Verification items for the finished model (mm, model axes). Give positions to 0.01 mm unless a question says otherwise; leave off trailing zeros. Order: outer loops, then holes, each group sorted by start corner. A loop starts at its lowest first (then second) coordinate and runs counter-clockwise, first axis right, second up.
from build123d import *

# Parameters (mm, degrees)
SKETCH001_W  = 54
SKETCH001_H  = 78
PAD001_DEPTH = 12
FILLET_R     = 2
FILLET001_R  = 2
SKETCH002_R  = 2
POCKET_DEPTH = 6
FILLET002_R  = 2


with BuildPart() as part:
    # Sketch001 (on Face1 of CopyCut) → Pad001 (new body)
    with BuildSketch(Plane.XY.offset(-3)):
        with Locations((0, 47)):
            Rectangle(SKETCH001_W, SKETCH001_H)
    extrude(amount=PAD001_DEPTH)

    # Fillet
    fillet_edges = [part.edges().sort_by_distance(p)[0] for p in [
        (0, 86, 9),
    ]]
    fillet(fillet_edges, radius=FILLET_R)

    # Fillet001
    fillet001_edges = [part.edges().sort_by_distance(p)[0] for p in [
        (-27, 46, 9),
        (27, 46, 9),
    ]]
    fillet(fillet001_edges, radius=FILLET001_R)

    # Sketch002 (on Face5 of Fillet001) → Pocket (cut)
    with BuildSketch(Plane(origin=(0, 0, -3), x_dir=(1, 0, 0), z_dir=(0, 0, -1))):
        with Locations((10, -70)):
            Circle(SKETCH002_R)
        with Locations((-10, -50)):
            Circle(SKETCH002_R)
    extrude(amount=-POCKET_DEPTH, mode=Mode.SUBTRACT)

    # Fillet002
    fillet002_edges = [part.edges().sort_by_distance(p)[0] for p in [
        (0, 8, 9),
    ]]
    fillet(fillet002_edges, radius=FILLET002_R)


solid = part.part
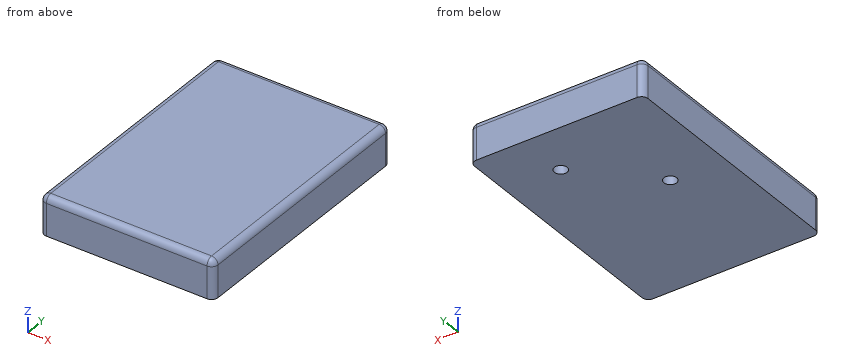
(1) Section check A-A, the plane y = 70. Enter the section's corners in (x, z).
Solved:
outline: (-27, -3) - (8, -3) - (8, 3) - (12, 3) - (12, -3) - (27, -3) - (27, 7) arc R2 ccw to (25, 9) - (-25, 9) arc R2 ccw to (-27, 7) - close
(2) Go/stop test with a flat-tipped pin: pin 1 (2 mm diameter, centred on x = 10.5, y = 69.5, fed in from -Z). Record where the tip stops, or that it passes through.
Solved:
pin 1: stops at z = 3
(3) Scan lines: line 1 (X direction, y = 50, z = -0.35); line 2 (X direction, y = 70, z = -0.85); line 3 (Y direction, x = 10, z = -0.5). Record each from-to range of solid material in increasing order.
Solved:
line 1: x = -27 to -12, -8 to 27
line 2: x = -27 to 8, 12 to 27
line 3: y = 8 to 68, 72 to 86
(4) Section check B-B, the plane x = -10. Enter the section's corners in (y, z), then the cut area to 3 significant figures.
Solved:
outline: (8, -3) - (48, -3) - (48, 3) - (52, 3) - (52, -3) - (86, -3) - (86, 7) arc R2 ccw to (84, 9) - (10, 9) arc R2 ccw to (8, 7) - close
area: 910 mm2
